Read the model definition and answer for the solid it produces. Units are mm, in the model's axes. Round coordinates to 2 decimals unless told otherwise and drop trailing zeros.
from build123d import *

# Parameters (mm, degrees)
BOSS_EXTRUDE1_DEPTH = 228.6


with BuildPart() as part:
    # Sketch1 → Boss-Extrude1 (new body)
    with BuildSketch(Plane.XY):
        with BuildLine():
            Line((-151.308507478, 320.448347343), (-153.902884159, 320.448347343))
            add(Edge.make_bspline(
                [(-153.902884159, 320.448347343), (-204.193593484, 355.830302978), (-209.681982797, 419.080625746)],
                knots=[0, 0, 0, 1, 1, 1], degree=2))
            add(Edge.make_bspline(
                [(-209.681982797, 419.080625746), (-212.468971889, 435.635081793), (-230.146422985, 426.26627389)],
                knots=[0, 0, 0, 1, 1, 1], degree=2))
            Line((-230.146422985, 426.26627389), (-254.364738426, 310.76353871))
            Line((-254.364738426, 310.76353871), (-260.02419987, 304.566542475))
            Line((-260.02419987, 304.566542475), (-258.578921486, 290.691869988))
            Line((-258.578921486, 290.691869988), (-265.193093483, 282.384698892))
            Line((-265.193093483, 282.384698892), (-263.369961518, 264.24078968))
            Line((-263.369961518, 264.24078968), (-272.846204191, 253.680341164))
            Line((-272.846204191, 253.680341164), (-273.030336503, 238.665049502))
            Line((-273.030336503, 238.665049502), (-279.067580784, 231.420751471))
            Line((-279.067580784, 231.420751471), (-278.892342657, 213.438930008))
            Line((-278.892342657, 213.438930008), (-285.037056209, 201.886868531))
            Line((-285.037056209, 201.886868531), (-285.631103618, 184.685583339))
            add(Edge.make_bspline(
                [(-285.631103618, 184.685583339), (-268.062935634, 203.22280378), (-246.614344295, 189.659725427)],
                knots=[0, 0, 0, 1, 1, 1], degree=2))
            add(Edge.make_bspline(
                [(-246.614344295, 189.659725427), (-127.920705679, 114.429612695), (6.673773744, 73.083350339)],
                knots=[0, 0, 0, 1, 1, 1], degree=2))
            add(Edge.make_bspline(
                [(6.673773744, 73.083350339), (28.666663993, 69.758079655), (50.443660227, 75.311339463)],
                knots=[0, 0, 0, 1, 1, 1], degree=2))
            add(Edge.make_bspline(
                [(50.443660227, 75.311339463), (77.641446166, 82.046433693), (104.763627465, 73.083350339)],
                knots=[0, 0, 0, 1, 1, 1], degree=2))
            add(Edge.make_bspline(
                [(104.763627465, 73.083350339), (141.460227891, 63.748172731), (179.63636286, 64.622561677)],
                knots=[0, 0, 0, 1, 1, 1], degree=2))
            Line((179.63636286, 64.622561677), (392.082197073, 58.29218063))
            add(Edge.make_bspline(
                [(392.082197073, 58.29218063), (482.5670898, 63.486005848), (568.127479803, 92.380936595)],
                knots=[0, 0, 0, 1, 1, 1], degree=2))
            add(Edge.make_bspline(
                [(568.127479803, 92.380936595), (595.430658845, 98.233924977), (619.963244193, 110.663717217)],
                knots=[0, 0, 0, 1, 1, 1], degree=2))
            add(Edge.make_bspline(
                [(619.963244193, 110.663717217), (629.007847964, 139.298696012), (606.486634537, 165.008668656)],
                knots=[0, 0, 0, 1, 1, 1], degree=2))
            add(Edge.make_bspline(
                [(606.486634537, 165.008668656), (580.79478885, 183.685281275), (550.927071991, 194.234435924)],
                knots=[0, 0, 0, 1, 1, 1], degree=2))
            add(Edge.make_bspline(
                [(550.927071991, 194.234435924), (500.725829633, 209.711245508), (449.760265594, 222.422706898)],
                knots=[0, 0, 0, 1, 1, 1], degree=2))
            add(Edge.make_bspline(
                [(449.760265594, 222.422706898), (241.262282516, 291.708486768), (60.192619276, 419.080625746)],
                knots=[0, 0, 0, 1, 1, 1], degree=2))
            add(Edge.make_bspline(
                [(60.192619276, 419.080625746), (24.832715259, 442.475671603), (-13.561949274, 460.190317475)],
                knots=[0, 0, 0, 1, 1, 1], degree=2))
            add(Edge.make_bspline(
                [(-13.561949274, 460.190317475), (-19.66491685, 459.046402337), (-17.821966678, 452.380802052)],
                knots=[0, 0, 0, 1, 1, 1], degree=2))
            add(Edge.make_bspline(
                [(-17.821966678, 452.380802052), (-12.318595056, 427.744919978), (-4.138222221, 403.861238748)],
                knots=[0, 0, 0, 1, 1, 1], degree=2))
            add(Edge.make_bspline(
                [(-4.138222221, 403.861238748), (1.674072586, 384.699876217), (-8.164307919, 366.08094882)],
                knots=[0, 0, 0, 1, 1, 1], degree=2))
            add(Edge.make_bspline(
                [(-8.164307919, 366.08094882), (-21.973615339, 326.401145795), (-61.04518825, 306.862929248)],
                knots=[0, 0, 0, 1, 1, 1], degree=2))
            add(Edge.make_bspline(
                [(-61.04518825, 306.862929248), (-108.230426593, 268.595120107), (-151.308507478, 320.448347343)],
                knots=[0, 0, 0, 1, 1, 1], degree=2))
        make_face()
    extrude(amount=BOSS_EXTRUDE1_DEPTH)


solid = part.part
Q1. Flat-ended cylindrical pins translate along their axes: pin 1 Ø2 at (x, z) = (-152.5, 154) entering from +Y; pin 2 Ø1.5 at (x, y) = (507.5, 115) entering from -Z; pin 3 Ø3 at (x, z) = (234.5, 102) entering from -Y; pin 4 Ø2 at (y, z) = (273.5, 78.5) entering from -X. Find the tip coordinate at first contact, or state that the pin passes through.
Verdict:
pin 1: stops at y = 320.45
pin 2: stops at z = 0
pin 3: stops at y = 62.94
pin 4: stops at x = -264.4
Q2. Determine the mould class of faces 1 (the flat face through (165, 217, 0)), 2 (the flat face through (-264.294, 273.44, 112.7)), 3 (the flat face through (-242.086, 369.323, 112.7)) for opening direction Y: pulls with the +Y half, pulls with the -Y half, needs draft (parallel to the pull), parting line crosses it, or undercut.
Verdict:
face 1: needs draft
face 2: undercut
face 3: pulls with the +Y half
Q3. Straight lines are drawn through the part: probe 1 along X at (y, z) = (413, 72); probe 2 along Y at (x, z) = (236.5, 85); probe 3 along Y at (x, z) = (-97.5, 122.5). For each, find the intervals that lie inside material, in ascending order.
Verdict:
probe 1: x = -232.93 to -209.04, -7.16 to 68.9
probe 2: y = 62.93 to 312.16
probe 3: y = 111.17 to 290.7
